Verification items for the finished model (mm, model axes). A direction names the side the tool comes from. Coordinates: 2 decimals unless noted, no trailing zeros. Order: outer loops, then holes, each group sorted by start corner. A loop starts at its lowest first (then second) coordinate and runs counter-clockwise, first axis right, second up. Notation, with made-up numbers: (79.25, -28) -> (98.25, -28) arc R17 cw to (98.25, -17) -> close; hole circle Ø10 at (71.5, 89). An arc over 180 degrees is marked (long way). Answer as CSV lines item,"result".
```python
from build123d import *

# Parameters (mm, degrees)
SKETCH1_R           = 25.4
BOSS_EXTRUDE1_DEPTH = 3.175


with BuildPart() as part:
    # Sketch1 → Boss-Extrude1 (new body)
    with BuildSketch(Plane(origin=(0, 0, 0), x_dir=(1, 0, 0), z_dir=(0, 1, 0))):
        with Locations(Location((0, 0, 0), (0, 0, 270))):
            Circle(SKETCH1_R)
        with BuildLine():
            Line((-2.919571886, 3.81), (-2.919571886, -3.81))
            ThreePointArc((-2.919571886, -3.81), (0, -4.8), (2.919571886, -3.81))
            Line((2.919571886, -3.81), (2.919571886, 3.81))
            ThreePointArc((2.919571886, 3.81), (0, 4.8), (-2.919571886, 3.81))
        make_face(mode=Mode.SUBTRACT)
    extrude(amount=-BOSS_EXTRUDE1_DEPTH)


solid = part.part
```
Item 1: Tool access check on faces 1 (the flat face through (0, 0, 5)), 2 (the cylindrical face through (0, -1.6, 4.8)). Record the directions out of +Z, -Z, +X, -X, +Y, -Y that give a thin tool (end or side, any length) a straight path to the whole face; none if there is none.
Answer list:
face 1,"+Z, -Z, +X, -X, +Y"
face 2,"+Y, -Y"
Item 2: Section check C-C, the plane y = -1.05. Record the boundary of the cut face in (x, z), plus the area to 3 significant figures.
Answer list:
outline,"circle Ø50.8 at (0, 0); hole (-2.92, -3.81) arc R4.8 ccw to (2.92, -3.81) -> (2.92, 3.81) arc R4.8 ccw to (-2.92, 3.81) -> close"
area,"1,970 mm2"
Item 3: Section check B-B, the plane z = 0. Record the boundary of the cut face in (x, y) (3 decimals), plus the area to 3 significant figures.
Answer list:
outline,"(-25.4, -3.175) -> (-2.92, -3.175) -> (-2.92, 0) -> (-25.4, 0) -> close; (2.92, -3.175) -> (25.4, -3.175) -> (25.4, 0) -> (2.92, 0) -> close"
area,"143 mm2"
Item 4: Section check D-D, the plane x = 20. Record the boundary of the cut face in (y, z) (3 decimals), plus the area to 3 significant figures.
Answer list:
outline,"(-3.175, -15.658) -> (0, -15.658) -> (0, 15.658) -> (-3.175, 15.658) -> close"
area,"99.4 mm2"
Item 5: Depth check by flat-ended pin: pin 1 Ø1.5 at (x, y) = (-15, -1.5) entering from +Z; pin 2 Ø1.5 at (y, z) = (-1, 18.5) entering from +X; pin 3 Ø1.5 at (y, z) = (-2.5, -5.5) entering from +X. Enter the tip coordinate at first touch or a pass-through.
Answer list:
pin 1,"z = 21.03"
pin 2,"x = 18.17"
pin 3,"x = 24.95"
Item 6: Section check A-A, the plane x = 0. Record the boundary of the cut face in (y, z) (3 decimals), plus the area to 3 significant figures.
Answer list:
outline,"(-3.175, -25.4) -> (0, -25.4) -> (0, -4.8) -> (-3.175, -4.8) -> close; (-3.175, 4.8) -> (0, 4.8) -> (0, 25.4) -> (-3.175, 25.4) -> close"
area,"131 mm2"
Item 7: Thickness scan on line 1 (Z direction, x = -1, y = -1.6); line 2 (X direction, y = -2, z = 1); line 3 (Z direction, x = -2, y = -2.9). Record the ranges inside material, lowest first.
Answer list:
line 1,"-25.38 to -4.69, 4.69 to 25.38"
line 2,"-25.38 to -2.92, 2.92 to 25.38"
line 3,"-25.32 to -4.36, 4.36 to 25.32"
Item 8: Release check for a two-part mould opening along Z. For faces 3 (the flat face through (0, -3.175, 5)), 4 (the cylindrical face through (-15.456, -1.565, -20.157)), 5 (the flat face through (-2.92, -2, 0)), 6 (the flat face through (2.92, -2, 0)) record: +Z half, -Z half, draft (parallel to the pull), parting line (faces both ways), or undercut.
Answer list:
face 3,"draft"
face 4,"parting line"
face 5,"undercut"
face 6,"undercut"
